```python
from build123d import *

# Parameters (mm, degrees)
SKETCH1_R         = 3.048
EXTRUDE1_DEPTH    = 8.89
CHAMFER1_SIZE     = 1.27
EXTRUDE2_DEPTH    = 3.81
SKETCH3_R         = 2.029785207
EXTRUDE3_DEPTH    = 1.27
SKETCH4_R         = 3.175
EXTRUDE4_DEPTH    = 1.27
DOME1_FACE_RADIUS = 3.175
DOME1_HEIGHT      = 2.54
FILLET1_R         = 1.27


with BuildPart() as part:
    # Sketch1 → Extrude1 (new body)
    with BuildSketch(Plane.XY):
        Circle(SKETCH1_R)
    extrude(amount=EXTRUDE1_DEPTH)

    # Chamfer1
    chamfer1_edges = [part.edges().sort_by_distance(p)[0] for p in [
        (-3.048, 0, 8.89),
    ]]
    chamfer(chamfer1_edges, length=CHAMFER1_SIZE)

    # Sketch2 → Extrude2 (add)
    with BuildSketch(Plane(origin=(0, 0, 0), x_dir=(-1, 0, 0), z_dir=(0, 0, -1))):
        Polygon((6.598292207, 0.104115064), (3.208979813, 5.766346205), (-3.389312394, 5.662231141), (-6.598292207, -0.104115064), (-3.208979813, -5.766346205), (3.389312394, -5.662231141), align=None)
    extrude(amount=EXTRUDE2_DEPTH)

    # Sketch3 → Extrude3 (add)
    with BuildSketch(Plane(origin=(0, 0, -3.81), x_dir=(-1, 0, 0), z_dir=(0, 0, -1))):
        Circle(SKETCH3_R)
    extrude(amount=EXTRUDE3_DEPTH)

    # Sketch4 → Extrude4 (add)
    with BuildSketch(Plane(origin=(0, 0, -5.08), x_dir=(-1, 0, 0), z_dir=(0, 0, -1))):
        Circle(SKETCH4_R)
    extrude(amount=EXTRUDE4_DEPTH)

    # Dome1: a dome of height H over a round flat face of radius A is a cap of a sphere of radius (A * A + H * H) / (2 * H)
    dome1_r = (DOME1_FACE_RADIUS * DOME1_FACE_RADIUS + DOME1_HEIGHT * DOME1_HEIGHT) / (2 * DOME1_HEIGHT)
    dome1_base = Plane((0, 0, -6.35), z_dir=(0, 0, -1))
    with Locations(dome1_base.offset(DOME1_HEIGHT - dome1_r)):
        dome1_ball = Sphere(dome1_r, mode=Mode.PRIVATE)
    add(split(dome1_ball, bisect_by=dome1_base, keep=Keep.TOP, mode=Mode.PRIVATE))

    # Fillet1
    fillet1_edges = [part.edges().sort_by_distance(p)[0] for p in [
        (3.389312394, 5.662231141, -1.905),
        (6.598292207, -0.104115064, -1.905),
        (3.208979813, -5.766346205, -1.905),
        (-4.993802301, -2.779058038, -3.81),
        (-4.90363601, 2.935230635, -3.81),
        (0.090166291, 5.714288673, -3.81),
        (4.993802301, 2.779058038, -3.81),
        (4.90363601, -2.935230635, -3.81),
        (-0.090166291, -5.714288673, -3.81),
        (-3.389312394, -5.662231141, -1.905),
        (-6.598292207, 0.104115064, -1.905),
        (-3.208979813, 5.766346205, -1.905),
    ]]
    fillet(fillet1_edges, radius=FILLET1_R)


solid = part.part
```
The listing builds one solid part. Answer for the finished solid, in the listing's coordinates (mm). A direction names the side the tool comes from. Coordinates: 2 decimals unless noted, no trailing zeros. Loops run counter-clockwise (first coordinate to the right, second up) from the corner with the lowest first, then second, coordinate; pieces in that order, holes last. Notation, with made-up numbers: (79, -2.75) - (102, -2.75) arc R20 cw to (102, 6.25) - close; hole circle Ø11 at (69, 18). An arc over 180 degrees is marked (long way). Use a Markdown table: item, result. Add a question column.
1) The part is cut by section C-C, the plane z = 1.25. Give the vertices of the cut face in (x, y).
2) The part is cut by section B-B, the plane z = -4.5. Give the vertices of the cut face in (x, y).
3) Given pin 1 (3 mm diameter, centred on x = -4.5, z = -1, fed in from -Y); pin 2 (2 mm diameter, centred on x = 4, y = -2, fed in from +Z); pin 3 (4 mm diameter, centred on x = 0, z = -1.5, fed in from +Y), each flat-ended and moving along its own axis, determine where each tip first touches the part or whether it passes through.
4) The mould has two halves that part along Z. Classify faces 6 (the flat face through (-1, -2, -5.08)), 7 (the flat face through (4.976, 2.81, -1.252)), 8 (the cylindrical face through (-4.678, -2.562, -3.448)), 9 (the cylindrical face through (0.264, 2.013, -4.436)): released by +Z, released by -Z, zero draft, split by the parting line, or undercut.
5) Find the intervals of material crossed by line 1 (Y direction, x = 0, z = 2.75); line 2 (Z direction, x = 3, y = -2); line 3 (X direction, y = 1.5, z = 2.25), in increasing order.
6) The part is cut by section A-A, the plane z = -2.25. Give the vertices of the cut face in (x, y).
7) For faces 1 (the flat face through (-2.2, 0.1, -3.81)), 2 (the cylindrical face through (-4.557, 2.77, -3.448)), 3 (the cylindrical face through (-3.296, -5.489, -1.288)), 4 (the flat face through (2.9, 1.4, 0)), 5 (the cylindrical face through (-0.12, -5.33, -3.45)), determine the directions among +Z, -Z, +X, -X, +Y, -Y from which every point of the face is accessible in a straight line to the end or side of a thin tool.
Here are the results:
| question | item | result |
|---|---|---|
| 1 | outline | circle Ø6.1 at (0, 0) |
| 2 | outline | circle Ø4.06 at (0, 0) |
| 3 | pin 1 | stops at y = -5.62 |
| 3 | pin 2 | stops at z = 0 |
| 3 | pin 3 | stops at y = 5.75 |
| 4 | face 6 | undercut |
| 4 | face 7 | zero draft |
| 4 | face 8 | released by -Z |
| 4 | face 9 | undercut |
| 5 | line 1 | y = -3.05 to 3.05 |
| 5 | line 2 | z = -3.81 to 0 |
| 5 | line 3 | x = -2.65 to 2.65 |
| 6 | outline | (-6.24, -0.54) - (-3.75, -5.02) arc R1.27 ccw to (-2.66, -5.67) - (2.48, -5.75) arc R1.27 ccw to (3.59, -5.14) - (6.22, -0.73) arc R1.27 ccw to (6.24, 0.54) - (3.75, 5.02) arc R1.27 ccw to (2.66, 5.67) - (-2.48, 5.75) arc R1.27 ccw to (-3.59, 5.14) - (-6.22, 0.73) arc R1.27 ccw to start |
| 7 | face 1 | none |
| 7 | face 2 | -Z, -X, +Y |
| 7 | face 3 | +Z, -Z, -X, -Y |
| 7 | face 4 | +Z |
| 7 | face 5 | -Z, -X, -Y |
